Input: part model. Units: mm. Frame: model coordinates. Coordinates: 2 decimals unless noted, no trailing zeros. Order: outer loops, then holes, each group sorted by start corner. A loop starts at its lowest first (then second) coordinate and runs counter-clockwise, first axis right, second up. Notation, with made-up numbers: M -34.75,-18.75 L 18.25,-18.75 A20 ccw 18.25,-6.75 Z; hole C 40.25,83.5 d4. An arc over 180 degrees is marked long. One line per item, written item: value.
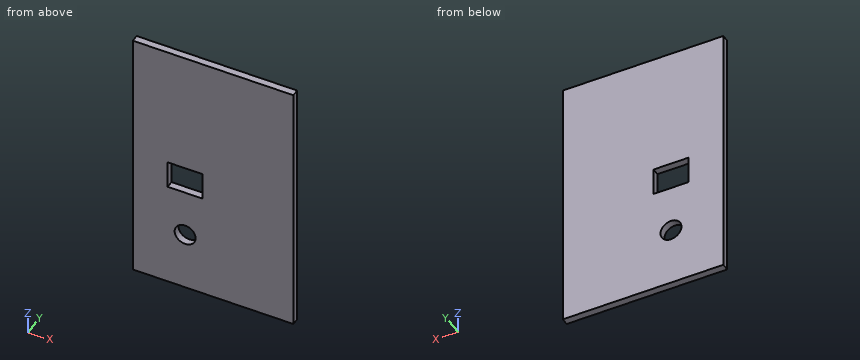
```python
from build123d import *

# Parameters (mm, degrees)
SKETCH1_W           = 23.005
SKETCH1_H           = 37.5
SKETCH1_R           = 1.5025
SKETCH1_W_2         = 5.005
SKETCH1_H_2         = 4.005
BOSS_EXTRUDE1_DEPTH = 1.05


with BuildPart() as part:
    # Sketch1 → Boss-Extrude1 (new body)
    with BuildSketch(Plane(origin=(0, 0, 0), x_dir=(1, 0, 0), z_dir=(0, 1, 0))):
        Rectangle(SKETCH1_W, SKETCH1_H)
        with Locations((-4.0025, 10.14275)):
            Circle(SKETCH1_R, mode=Mode.SUBTRACT)
        with Locations((-4, 1.2525)):
            Rectangle(SKETCH1_W_2, SKETCH1_H_2, mode=Mode.SUBTRACT)
    extrude(amount=BOSS_EXTRUDE1_DEPTH)


solid = part.part
```
(1) First-contact query: pin 1 (5 mm diameter, centred on x = -8.5, z = 14.5, fed in from -Y). Flat tip, straight axial feed; report the tip coordinate or a pass-through.
Data:
pin 1: stops at y = 0
(2) Ray query, line 1 (X direction, y = 0.1, z = -10); line 2 (Z direction, x = -6, y = 0.55) (3 decimals); line 3 (Z direction, x = -4.25, y = 0.35) (3 decimals). Return the intervals inside material, ascending. Write a range as from..to.
Data:
line 1: x = -11.5..-5.5, -2.51..11.5
line 2: z = -18.75..-3.255, 0.75..18.75
line 3: z = -18.75..-11.625, -8.661..-3.255, 0.75..18.75
(3) Cut plane A-A on z = 0. Output: boundary loops of the cut face in (x, y), plus the area to 3 significant figures.
Data:
outline: M -11.5,0 L -6.5,0 L -6.5,1.05 L -11.5,1.05 Z; M -1.5,0 L 11.5,0 L 11.5,1.05 L -1.5,1.05 Z
area: 18.9 mm2
(4) Cut plane B-B on y = 0.65. Give the number of separate pieces and of enclosed holes in the cut face, plus the area to 3 significant figures.
Data:
separate pieces: 1
enclosed holes: 2
area: 836 mm2
(5) Cut plane C-C on z = -9. Output: boundary loops of the cut face in (x, y), plus the area to 3 significant figures.
Data:
outline: M -11.5,0 L -4.98,0 L -4.98,1.05 L -11.5,1.05 Z; M -3.03,0 L 11.5,0 L 11.5,1.05 L -3.03,1.05 Z
area: 22.1 mm2
